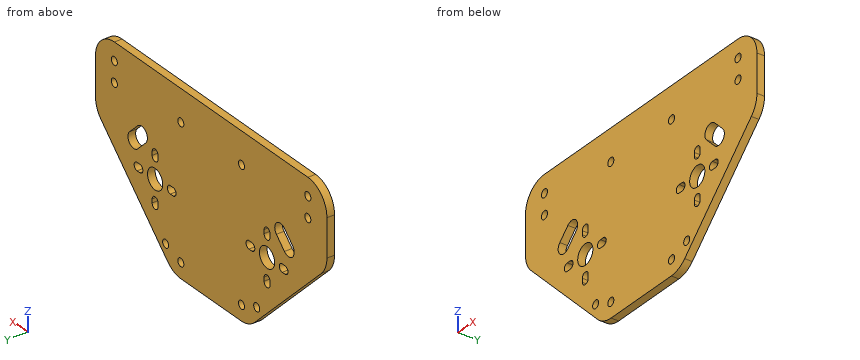
from build123d import *

# Parameters (mm, degrees)
EXTRUDE_1_DEPTH     = 3
SKETCH_2_R          = 1.6
SKETCH_2_R_2        = 4
CUT_EXTRUDE_1_DEPTH = 3


with BuildPart() as part:
    # 草图1 → 凸台-拉伸1 (new body)
    with BuildSketch(Plane(origin=(0, 0, 0), x_dir=(1, 0, 0), z_dir=(0, 1, 0))):
        with BuildLine():
            Line((0, 30), (-15.857864376, 30))
            ThreePointArc((-15.857864376, 30), (-19.6846987, 29.238795325), (-22.928932188, 27.071067812))
            Line((-22.928932188, 27.071067812), (-58.071067812, -8.071067812))
            ThreePointArc((-58.071067812, -8.071067812), (-60.238795325, -11.3153013), (-61, -15.142135624))
            Line((-61, -15.142135624), (-61, -30.000000004))
            ThreePointArc((-61, -30.000000004), (-58.071067812, -37.071067816), (-51, -40.000000004))
            Line((-51, -40.000000004), (-36, -40.000000004))
            Line((-36, -40.000000004), (36, -40.000000004))
            Line((36, -40.000000004), (51, -40.000000004))
            ThreePointArc((51, -40.000000004), (58.071067812, -37.071067816), (61, -30.000000004))
            Line((61, -30.000000004), (61, -15.142135624))
            ThreePointArc((61, -15.142135624), (60.238795325, -11.3153013), (58.071067812, -8.071067812))
            Line((58.071067812, -8.071067812), (22.928932188, 27.071067812))
            ThreePointArc((22.928932188, 27.071067812), (19.6846987, 29.238795325), (15.857864376, 30))
            Line((15.857864376, 30), (0, 30))
        make_face()
    extrude(amount=EXTRUDE_1_DEPTH)

    # 草图2 → 切除-拉伸1 (cut)
    with BuildSketch(Plane(origin=(0, 0, 0), x_dir=(1, 0, 0), z_dir=(0, 1, 0))):
        with Locations(Location((-16, 24, 0), (0, 0, 270))):
            Circle(SKETCH_2_R)
        with Locations(Location((16, 24, 0), (0, 0, 270))):
            Circle(SKETCH_2_R)
        with Locations(Location((-24, 21, 0), (0, 0, 270))):
            Circle(SKETCH_2_R)
        with Locations(Location((24, 21, 0), (0, 0, 270))):
            Circle(SKETCH_2_R)
        with Locations(Location((-29.450477816, 0, 0), (0, 0, 270))):
            Circle(SKETCH_2_R_2)
        with Locations(Location((29.549522184, 0, 0), (0, 0, 90))):
            Circle(SKETCH_2_R_2)
        with Locations(Location((-50.950477816, -25, 0), (0, 0, 270))):
            Circle(SKETCH_2_R)
        with Locations(Location((-50.950477816, -33, 0), (0, 0, 270))):
            Circle(SKETCH_2_R)
        with Locations(Location((51.049522184, -33, 0), (0, 0, 90))):
            Circle(SKETCH_2_R)
        with Locations(Location((51.049522184, -25, 0), (0, 0, 90))):
            Circle(SKETCH_2_R)
        with Locations(Location((-16, -27.5, 0), (0, 0, 270))):
            Circle(SKETCH_2_R)
        with Locations(Location((16, -27.5, 0), (0, 0, 270))):
            Circle(SKETCH_2_R)
        with BuildLine():
            Line((-37.450477816, -1.55), (-38.950477816, -1.55))
            ThreePointArc((-38.950477816, -1.55), (-40.500477816, 0), (-38.950477816, 1.55))
            Line((-38.950477816, 1.55), (-37.450477816, 1.55))
            ThreePointArc((-37.450477816, 1.55), (-35.900477816, 0), (-37.450477816, -1.55))
        make_face()
        with BuildLine():
            Line((38.728201841, -6.678679656), (34.485561154, -10.921320344))
            ThreePointArc((34.485561154, -10.921320344), (34.485561154, -15.163961031), (38.728201841, -15.163961031))
            Line((38.728201841, -15.163961031), (42.970842528, -10.921320344))
            ThreePointArc((42.970842528, -10.921320344), (42.970842528, -6.678679656), (38.728201841, -6.678679656))
        make_face()
        with BuildLine():
            Line((-31.000477816, 8), (-31.000477816, 9.5))
            ThreePointArc((-31.000477816, 9.5), (-29.450315952, 11.050161864), (-27.900154088, 9.5))
            Line((-27.900154088, 9.5), (-27.900154088, 8))
            ThreePointArc((-27.900154088, 8), (-29.450315952, 6.449838136), (-31.000477816, 8))
        make_face()
        with BuildLine():
            Line((-27.900477816, -8), (-27.900477816, -9.5))
            ThreePointArc((-27.900477816, -9.5), (-29.450477816, -11.05), (-31.000477816, -9.5))
            Line((-31.000477816, -9.5), (-31.000477816, -8))
            ThreePointArc((-31.000477816, -8), (-29.450477816, -6.45), (-27.900477816, -8))
        make_face()
        with BuildLine():
            Line((-21.450477816, 1.55), (-19.950477816, 1.55))
            ThreePointArc((-19.950477816, 1.55), (-18.400477816, 0), (-19.950477816, -1.55))
            Line((-19.950477816, -1.55), (-21.450477816, -1.55))
            ThreePointArc((-21.450477816, -1.55), (-23.000477816, 0), (-21.450477816, 1.55))
        make_face()
        with BuildLine():
            Line((21.549522184, -1.55), (20.049522184, -1.55))
            ThreePointArc((20.049522184, -1.55), (18.499522184, 0), (20.049522184, 1.55))
            Line((20.049522184, 1.55), (21.549522184, 1.55))
            ThreePointArc((21.549522184, 1.55), (23.099522184, 0), (21.549522184, -1.55))
        make_face()
        with BuildLine():
            Line((-42.871798159, -10.921320344), (-38.629157472, -15.163961031))
            ThreePointArc((-38.629157472, -15.163961031), (-34.386516785, -15.163961031), (-34.386516785, -10.921320344))
            Line((-34.386516785, -10.921320344), (-38.629157472, -6.678679656))
            ThreePointArc((-38.629157472, -6.678679656), (-42.871798159, -6.678679656), (-42.871798159, -10.921320344))
        make_face()
        with BuildLine():
            Line((31.099522184, -8), (31.099522184, -9.5))
            ThreePointArc((31.099522184, -9.5), (29.549522184, -11.05), (27.999522184, -9.5))
            Line((27.999522184, -9.5), (27.999522184, -8))
            ThreePointArc((27.999522184, -8), (29.549522184, -6.45), (31.099522184, -8))
        make_face()
        with BuildLine():
            Line((27.999522184, 8), (27.999522184, 9.5))
            ThreePointArc((27.999522184, 9.5), (29.549522184, 11.05), (31.099522184, 9.5))
            Line((31.099522184, 9.5), (31.099522184, 8))
            ThreePointArc((31.099522184, 8), (29.549522184, 6.45), (27.999522184, 8))
        make_face()
        with BuildLine():
            Line((37.549522184, 1.55), (39.049522184, 1.55))
            ThreePointArc((39.049522184, 1.55), (40.599522184, 0), (39.049522184, -1.55))
            Line((39.049522184, -1.55), (37.549522184, -1.55))
            ThreePointArc((37.549522184, -1.55), (35.999522184, 0), (37.549522184, 1.55))
        make_face()
    extrude(amount=CUT_EXTRUDE_1_DEPTH, mode=Mode.SUBTRACT)


solid = part.part
For this review, take the finished solid that the model builds, in its own axes (mm). Give positions to 0.01 mm unless a question says otherwise; leave off trailing zeros. Loops run counter-clockwise (first coordinate to the right, second up) from the corner with the lowest first, then second, coordinate; pieces in that order, holes last. Notation, with made-up numbers: M -27,49 L 15,49 A19 cw 15,71 Z; hole C 81.25,85 d4. An arc over 180 degrees is marked long. Answer as a JSON object with one key per item and string values. Group by question number.
Q1. Add section C-C on x = 45. Give the boundary of the cut face in (y, z), and give its area (3 significant figures).
Q2. Add section A-A on z = -24. Give the boundary of the cut face in (x, y).
Q3. Add section D-D on y = 0.5. Give the number of separate pieces and of enclosed holes in the cut face, and give its area (3 significant figures).
Q4. Insertion check: P1, Ø0.8, axis at y = 2, z = -8.5, coming from the +X side; P2, Ø1.2, axis at y = 2, z = 9, coming from the -X side; P3, Ø1.2, axis at y = 1.5, z = -9, coming from the -X side. Each pin has a flat end and moves straight along its axis. Give the tip position at first contact, or say it passes through.
Q5. Add section B-B on z = -16.5. Give the boundary of the cut face in (x, y).
Q6. For probe 1 along X at (y, z) = (1.35, 27.5); probe 2 along X at (y, z) = (1.1, 25); probe 3 along Z at (x, y) = (-40, 0.85), list the stretches that pass through material, from the lowest coordinate up. Write a range as [from, to].
Checked values:
{
 "1": {"outline": "M 0,-5 L 3,-5 L 3,40 L 0,40 Z", "area": "135 mm²"},
 "2": {"outline": "M -26,0 L -17.6,0 L -17.6,3 L -26,3 Z; M -14.4,0 L 14.4,0 L 14.4,3 L -14.4,3 Z; M 17.6,0 L 26,0 L 26,3 L 17.6,3 Z"},
 "3": {"separate pieces": "1", "enclosed holes": "22", "area": "6,400 mm²"},
 "4": {"P1": "x = 41.9", "P2": "x = -59.32", "P3": "x = -41.6"},
 "5": {"outline": "M -33.5,0 L 33.5,0 L 33.5,3 L -33.5,3 Z"},
 "6": {"probe 1": "[-61, -17.6], [-14.4, 14.4], [17.6, 61]", "probe 2": "[-61, -52.55], [-49.35, 49.45], [52.65, 61]", "probe 3": "[-10, -1.14], [1.14, 5.9], [13.79, 40]"}
}
